Read the model definition and answer for the solid it produces. Units are mm, in the model's axes. Face numbers are marked on the shaded views. A direction names the side the tool comes from. Coordinates: 2 decimals unless noted, no trailing zeros. Order: outer loops, then holes, each group sorted by start corner. A loop starts at its lowest first (then second) coordinate and runs counter-clockwise, first axis right, second up. Notation, with made-up numbers: M 11.5,7.25 L 59.5,7.25 A27 cw 59.5,25.25 Z; hole C -33,85.25 d7. An arc over 180 degrees is marked long. Put each result on its own line as item: value.
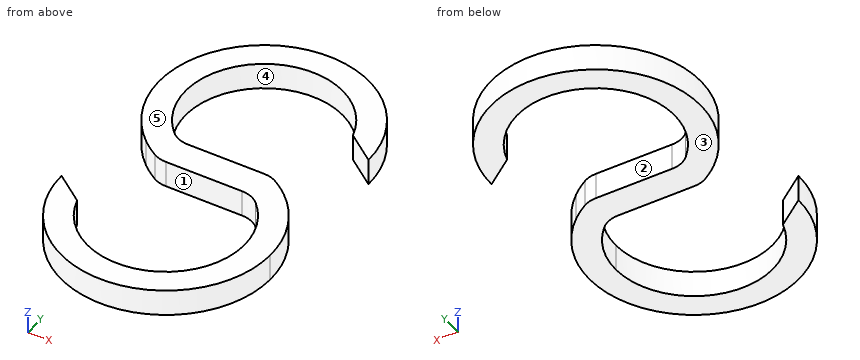
from build123d import *

# Parameters (mm, degrees)
F1_DEPTH    = 5
F2_T1_DEPTH = 31.594870106
F3_R        = 5


# Not quite as in the source:
# - a fillet or chamfer that OpenCascade refuses, or shapes differently, is made with other operations: its cross-section is extruded or revolved along the edge and cut away or added


with BuildPart() as f1:
    # F0 (on Top) → F1 (new body)
    with BuildSketch(Plane.XY):
        with BuildLine():
            ThreePointArc((20, 45), (-8.2287565553, 63.2287565553), (-13.2287565553, 30))
            ThreePointArc((-13.2287565553, 30), (-11.1540260033, 31.6008344344), (-8.8878037532, 32.9166666667))
            ThreePointArc((-8.8878037532, 32.9166666667), (-14.2521928137, 49.6770717335), (0, 60))
            ThreePointArc((0, 60), (10.6066017178, 55.6066017178), (15, 45))
            Line((15, 45), (20, 45))
        make_face()
        with BuildLine():
            ThreePointArc((-13.2287565553, 30), (-11.1540260033, 28.3991655656), (-8.8878037532, 27.0833333333))
            ThreePointArc((-8.8878037532, 27.0833333333), (-4.6770717335, 29.2521928137), (0, 30))
            ThreePointArc((0, 30), (-4.6770717335, 30.7478071863), (-8.8878037532, 32.9166666667))
            ThreePointArc((-8.8878037532, 32.9166666667), (-11.1540260033, 31.6008344344), (-13.2287565553, 30))
        make_face()
        with BuildLine():
            ThreePointArc((-8.8878037532, 32.9166666667), (-4.6770717335, 30.7478071863), (0, 30))
            Line((0, 30), (0, 32.9166666667))
            Line((0, 32.9166666667), (-8.8878037532, 32.9166666667))
        make_face()
        with BuildLine():
            ThreePointArc((0, 30), (-4.6770717335, 29.2521928137), (-8.8878037532, 27.0833333333))
            Line((-8.8878037532, 27.0833333333), (0, 27.0833333333))
            Line((0, 27.0833333333), (0, 30))
        make_face()
        with BuildLine():
            Line((0, 27.0833333333), (8.8878037532, 27.0833333333))
            ThreePointArc((8.8878037532, 27.0833333333), (4.6770717335, 29.2521928137), (0, 30))
            Line((0, 30), (0, 27.0833333333))
        make_face()
        with BuildLine():
            Line((0, 32.9166666667), (0, 30))
            ThreePointArc((0, 30), (4.6770717335, 30.7478071863), (8.8878037532, 32.9166666667))
            Line((8.8878037532, 32.9166666667), (0, 32.9166666667))
        make_face()
        with BuildLine():
            ThreePointArc((0, 30), (4.6770717335, 29.2521928137), (8.8878037532, 27.0833333333))
            ThreePointArc((8.8878037532, 27.0833333333), (11.1540260033, 28.3991655656), (13.2287565553, 30))
            ThreePointArc((13.2287565553, 30), (11.1540260033, 31.6008344344), (8.8878037532, 32.9166666667))
            ThreePointArc((8.8878037532, 32.9166666667), (4.6770717335, 30.7478071863), (0, 30))
        make_face()
        with BuildLine():
            ThreePointArc((15, 15), (10.6066017178, 4.3933982822), (0, 0))
            ThreePointArc((0, 0), (-10.6066017178, 4.3933982822), (-15, 15))
            Line((-15, 15), (-20, 15))
            ThreePointArc((-20, 15), (0, -5), (20, 15))
            ThreePointArc((20, 15), (18.2287565553, 23.2287565553), (13.2287565553, 30))
            ThreePointArc((13.2287565553, 30), (11.1540260033, 28.3991655656), (8.8878037532, 27.0833333333))
            ThreePointArc((8.8878037532, 27.0833333333), (13.3850113242, 21.7706330465), (15, 15))
        make_face()
    extrude(amount=F1_DEPTH)

    # F2: chamfer of 6 on 2 edges, made by hand

    # F2_s2 → F2_t1 (cut)
    with BuildSketch(Plane.XY.offset(-13.297435053)):
        with BuildLine():
            Line((-14.3747227125, 10.7142857143), (-20.1246117975, 15))
            Line((-20.1246117975, 15), (-15, 15))
            ThreePointArc((-15, 15), (-14.830161389, 12.7491527872), (-14.3747227125, 10.7142857143))
        make_face()
        with BuildLine():
            Line((20.1246117975, 45), (14.3747227125, 49.2857142857))
            ThreePointArc((14.3747227125, 49.2857142857), (14.830161389, 47.2508472128), (15, 45))
            Line((15, 45), (20.1246117975, 45))
        make_face()
    extrude(amount=F2_T1_DEPTH, mode=Mode.SUBTRACT)

    # F3
    f3_edges = [f1.edges().sort_by_distance(p)[0] for p in [
        (-8.887804, 32.916667, 2.5),
        (8.887804, 27.083333, 2.5),
        (8.887804, 32.916667, 2.5),
        (-8.887804, 27.083333, 2.5),
    ]]
    fillet(f3_edges, radius=F3_R)


solid = f1.part
Q1. A tool of negligible diameter and unlimited length cuts with its end or side. For the marked faces 1, 2 and 3, from which of +Z, -Z, +X, -X, +Y, -Y can it reach the whole face along a straight path? Write none if from no direction.
Answers below:
face 1: +Z, -Z, -X
face 2: +Z, -Z, +X
face 3: -Z, +X, -X, +Y, -Y
Q2. Find section D-D on x = 17. Write down the section's boundary in (y, z).
Answers below:
outline: M 4.46,0 L 25.54,0 L 25.54,5 L 4.46,5 Z; M 47.33,0 L 55.54,0 L 55.54,5 L 47.33,5 Z
Q3. Find section B-B on y = 3.5. Write down the section's boundary in (x, z), plus the area to 3 significant figures.
Answers below:
outline: M -16.36,0 L -9.63,0 L -9.63,5 L -16.36,5 Z; M 9.63,0 L 16.36,0 L 16.36,5 L 9.63,5 Z
area: 67.3 mm^2
Q4. Find section C-C on z = 1.5. Write down the section's boundary in (x, y) (3 decimals), plus the area to 3 significant figures.
Answers below:
outline: M -20,14.907 A20 ccw long 10.168,32.222 A5 ccw 7.626,32.917 L -7.059,32.917 A5 cw -10.588,34.375 A15 cw long 14.375,49.286 L 20,45.093 A20 ccw long -10.168,27.778 A5 ccw -7.626,27.083 L 7.059,27.083 A5 cw 10.588,25.625 A15 cw long -14.375,10.714 Z
area: 815 mm^2
Q5. Consider line 1 along Y through (x, z) = (0, 1.2); line 2 along Y through (x, z) = (7.5, 1.35); line 3 along X through (y, z) = (45, 4.05). Determine where each line is inside the solid, lowest interval first.
Answers below:
line 1: y = -5 to 0, 27.08 to 32.92, 60 to 65
line 2: y = -3.54 to 2.01, 27.06 to 32.92, 57.99 to 63.54
line 3: x = -20 to -15
Q6. For a pull along Y with two mould halves and no side action, classify the marked faces 4 and 5 as +Y half, -Y half, draft (parallel to the pull), parting line (faces both ways), or undercut.
Answers below:
face 4: undercut
face 5: draft
Q7. Find section A-A on x = 0. Write down the section's boundary in (y, z).
Answers below:
outline: M -5,0 L 0,0 L 0,5 L -5,5 Z; M 27.08,0 L 32.92,0 L 32.92,5 L 27.08,5 Z; M 60,0 L 65,0 L 65,5 L 60,5 Z
Q8. Given pin 1 (1 mm diameter, centred on y = 30, z = 3, fed in from +X) (3 decimals); pin 2 (1.5 mm diameter, centred on y = 5.5, z = 0.5, fed in from -X), each flat-ended and moving along its own axis, determine where each tip first touches the part or whether it passes through.
Answers below:
pin 1: stops at x = 13.775
pin 2: stops at x = -17.98
